Input: dimensioned drawing with shaded views. Units: mm. Origin: part minimum x, y, z. A direction names the side the tool comes from. Round coordinates to 2 decimals unless told otherwise and drop trailing zeros. Loops run counter-clockwise (first coordinate to the right, second up) from the corner with the lowest first, then second, coordinate; pieces in that order, holes last. Notation, with made-up numbers: (80, 80.5) -> (138, 80.5) arc R29 ccw to (138, 110.5) -> close; hole circle Ø3 at (17, 50). An arc over 180 degrees is marked (long way). Answer as a JSON object with one key per item and string values.
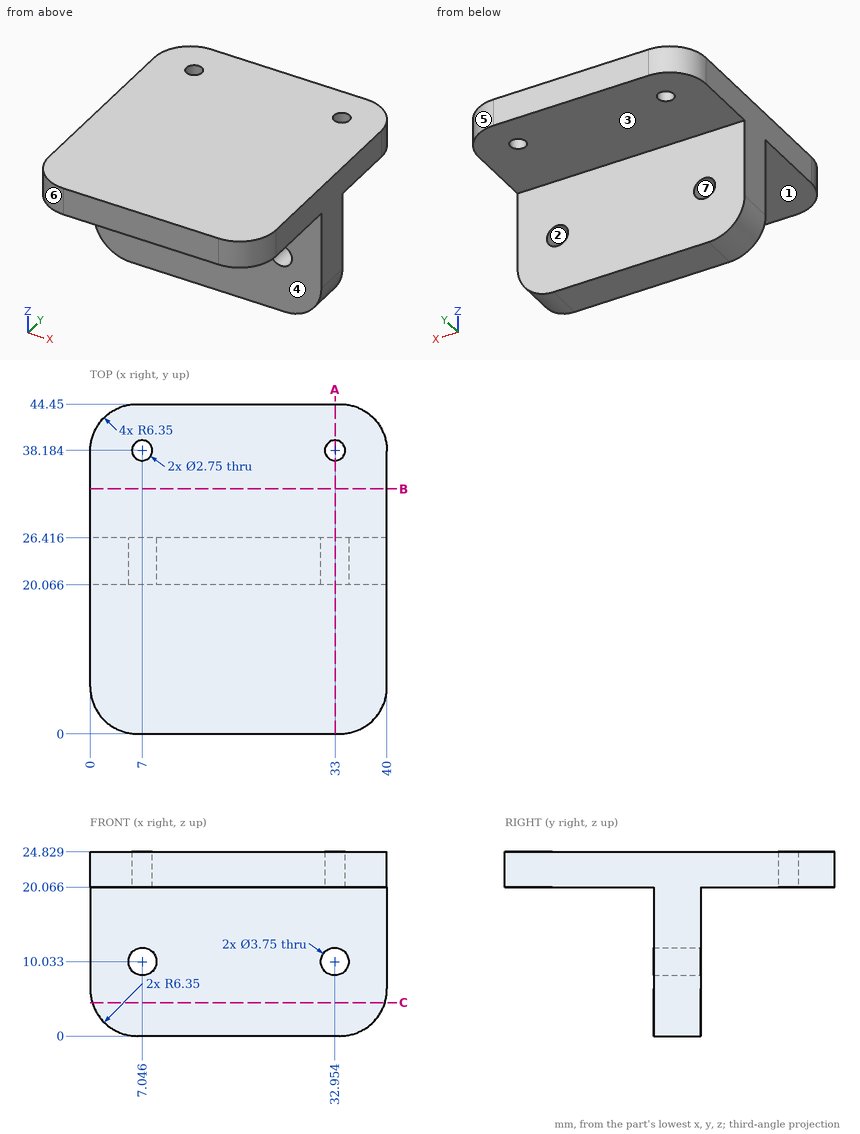
1) Contact query for flat-ended pins moving along their axis: P1, Ø6, axis at x = 34.5, z = 3, coming from the -Y side; P2, Ø9, axis at x = 12, y = 31.5, coming from the -Z side; P3, Ø2, axis at x = 32.954, z = 10.033, coming from the +Y side; P4, Ø2, axis at x = 20, z = 4.5, coming from the +Y side. Output: stop coordinate, or through.
Output:
{"P1": "stops at y = 20.07", "P2": "stops at z = 20.07", "P3": "passes through", "P4": "stops at y = 26.42"}
2) Reachability of the marked faces 1, 2 and 3 from +Z, -Z, +X, -X, +Y, -Y: full face, straight path, thin tool, end or side. Return the list, or none.
Output:
{"face 1": "-Z, +X, -X, -Y", "face 2": "+Y, -Y", "face 3": "-Z, +X, -X, +Y"}
3) Ray query, probe 1 along Y at (x, z) = (7, 23.2); probe 2 along Z at (x, y) = (30, 12) (1 decimal); probe 3 along Y at (x, z) = (20, 16.5) (1 decimal). Return the intervals inside material, ascending.
Output:
{"probe 1": "y = 0 to 36.81, 39.56 to 44.45", "probe 2": "z = 20.1 to 24.8", "probe 3": "y = 20.1 to 26.4"}
4) Section A-A, the plane x = 33. Count the separate pieces of the cut face and the enclosed holes in it, plus the area to 3 significant figures.
Output:
{"separate pieces": "3", "enclosed holes": "0", "area": "302 mm^2"}
5) Draft query along X for the marked faces 4, 5, 6 and 7. Return one class per face: +X half, -X half, draft (parallel to the pull), parting line (faces both ways), or undercut.
Output:
{"face 4": "draft", "face 5": "+X half", "face 6": "-X half", "face 7": "undercut"}
6) Section B-B, the plane y = 33. Output: boundary loops of the cut face in (x, z) (1 decimal).
Output:
{"outline": "(0, 20.1) -> (40, 20.1) -> (40, 24.8) -> (0, 24.8) -> close"}
7) Section C-C, the plane z = 4.5. Output: boundary loops of the cut face in (x, y) (1 decimal).
Output:
{"outline": "(0.3, 20.1) -> (39.7, 20.1) -> (39.7, 26.4) -> (0.3, 26.4) -> close"}
